Can you work these out from the model? Positions are in its coordinate system, mm. Coordinates: 2 decimals unless noted, no trailing zeros. Loops run counter-clockwise (first coordinate to the right, second up) from the corner with the lowest first, then second, coordinate; pieces in that order, holes last. Notation, with made-up numbers: (-7.75, 72) -> (-3.75, 72) arc R22 cw to (-3.75, 87) -> close; hole circle Ø8 at (29.5, -1). An arc over 180 degrees is marked (long way). Use one line per item in the form item = value. Start each with the question number.
(1) Imagine slicing it at A-A (x = 13). List the corners of the cut face in (y, z) for me (3 decimals).
(2) I need wall thicknesses on line 1 (Y direction, x = 9.25, z = 685.8); line 2 (Z direction, x = 13.5, y = 27); line 3 (Y direction, x = 17.5, z = 49.5). Which ranges of each line are inside material? Lowest first, please. Write a range as [from, to].
(3) I'm going to push a flat-ended pin straight in: pin 1 (5 mm diameter, centred on x = 7, y = 30.5, fed in from -Z). Where does the tip first touch, or does it pass through?
```python
from build123d import *

# Parameters (mm, degrees)
F0_W     = 19.05
F0_H     = 57.15
F1_DEPTH = 711.2
F2_W     = 19.05
F2_H     = 57.15
F3_DEPTH = 19.05
F4_R     = 3.302
F5_DEPTH = 19.05


with BuildPart() as f1:
    # F0 (on Top) → F1 (new body)
    with BuildSketch(Plane.XY):
        with Locations((9.525, 28.575)):
            Rectangle(F0_W, F0_H)
    extrude(amount=F1_DEPTH)

    # F2 (on face) → F3 (cut, through all)
    with BuildSketch(Plane.YZ.offset(19.05)):
        with Locations((28.575, 28.575)):
            Rectangle(F2_W, F2_H)
    extrude(amount=-F3_DEPTH, mode=Mode.SUBTRACT)

    # F4 (on face) → F5 (cut, through all)
    with BuildSketch(Plane(origin=(0, 0, 0), x_dir=(0, -1, 0), z_dir=(-1, 0, 0))):
        with Locations((-28.575, 685.8)):
            Circle(F4_R)
        with Locations((-28.575, 584.2)):
            Circle(F4_R)
    extrude(amount=-F5_DEPTH, mode=Mode.SUBTRACT)


solid = f1.part
```
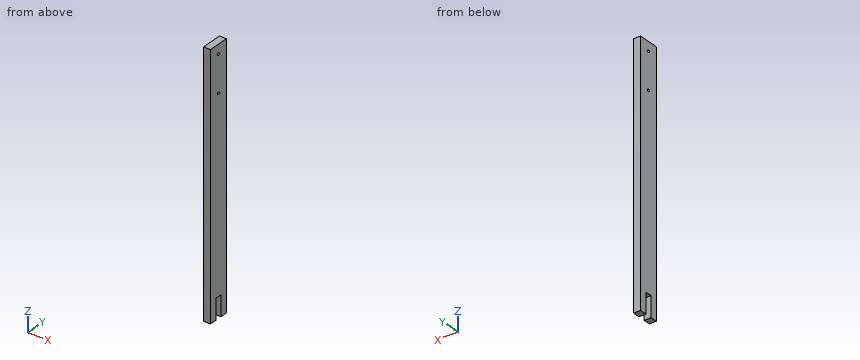
Worked out:
q1.outline = (0, 0) -> (19.05, 0) -> (19.05, 57.15) -> (38.1, 57.15) -> (38.1, 0) -> (57.15, 0) -> (57.15, 711.2) -> (0, 711.2) -> close; hole circle Ø6.604 at (28.575, 584.2); hole circle Ø6.604 at (28.575, 685.8)
q2.line_1 = [0, 25.27], [31.88, 57.15]
q2.line_2 = [57.15, 581.3], [587.1, 682.9], [688.7, 711.2]
q2.line_3 = [0, 19.05], [38.1, 57.15]
q3.pin_1 = 57.15
